Design review of the part built by this model. Coordinates are the model's own, in mm. Face numbers are marked on the shaded views. A direction names the side the tool comes from. Coordinates: 2 decimals unless noted, no trailing zeros. Write each loop counter-clockwise with the first axis right and the second up, starting at its lowest first coordinate (ties: lowest second). Pieces come first, ordered by that corner, then holes. Notation, with made-up numbers: (-38, 5.25) - (4, 5.25) arc R29 ccw to (4, 38.25) - close; hole circle Ø5 at (31, 29.25). An arc over 180 degrees is marked (long way). Use a Markdown table: item, result.
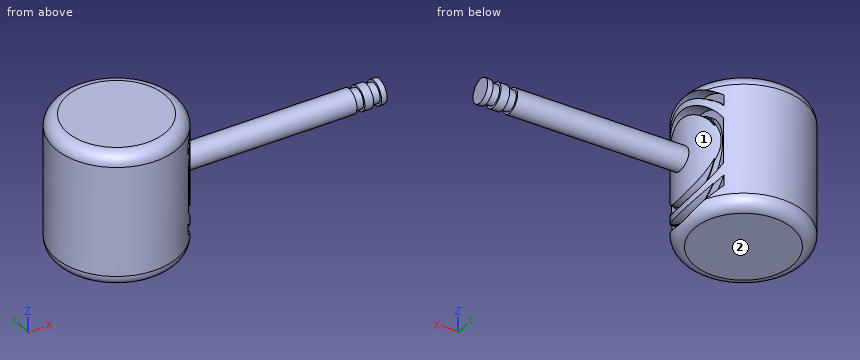
from build123d import *

# Parameters (mm, degrees)
F0_W   = 25.4
F0_H   = 55.7187045847
F2_W   = 118.6923170462
F2_H   = 4.8982012086
F4_W   = 3.185287118
F4_H   = 12.2274383903
F4_W_2 = 20.8224356174
F4_H_2 = 3.0317753553


# Not quite as in the source:
# - a fillet or chamfer that OpenCascade refuses, or shapes differently, is made with other operations: its cross-section is extruded or revolved along the edge and cut away or added


with BuildPart() as f1:
    # F0 (on Front) → F1 (revolve)
    with BuildSketch(Plane.XZ):
        Rectangle(F0_W, F0_H)
    revolve(axis=Axis((12.7, 0, 0), (0, 0, -1)))

    # F2 (on Front) → F3 (revolve)
    with BuildSketch(Plane.XZ):
        with Locations((59.3461585231, -2.4491006043)):
            Rectangle(F2_W, F2_H)
    revolve(axis=Axis((59.3461585231, 0, 0), (-1, 0, 0)))

    # F4 (on Front) → F6 (revolve, cut)
    with BuildSketch(Plane.XZ):
        with Locations((114.8856207728, -10.0567732006)):
            Rectangle(F4_W, F4_H)
        with Locations((108.191460371, -10.1317744702)):
            Rectangle(F4_W, F4_H)
        with Locations((43.9788103104, -24.0039676428)):
            Rectangle(F4_W_2, F4_H_2)
        with Locations((43.7408648431, -17.8672224283)):
            Rectangle(F4_W_2, F4_H_2)
        with Locations((41.584610939, 18.3283146471)):
            Rectangle(F4_W_2, F4_H_2)
        with Locations((41.4398871362, 24.3011359125)):
            Rectangle(F4_W_2, F4_H_2)
    revolve(axis=Axis((52.5897778571, 0, 0), (1, 0, 0)), mode=Mode.SUBTRACT)

    # F7: fillet of radius 5 on 1 edges, made by hand

    # F7_s1 → F7_t2 (revolve, cut)
    with BuildSketch(Plane.XZ):
        with BuildLine():
            ThreePointArc((-12.7, -22.8593522923), (-11.2355339059, -26.3948861983), (-7.7, -27.8593522923))
            Line((-7.7, -27.8593522923), (-12.7, -27.8593522923))
            Line((-12.7, -27.8593522923), (-12.7, -22.8593522923))
        make_face()
    revolve(axis=Axis((12.7, 0, -27.8593522923), (0, 0, -1)), mode=Mode.SUBTRACT)

    # F8: fillet of radius 5 on 1 edges, made by hand

    # F8_s1 → F8_t2 (revolve, cut)
    with BuildSketch(Plane.XZ):
        with BuildLine():
            ThreePointArc((-7.7, 27.8593522923), (-11.2355339059, 26.3948861983), (-12.7, 22.8593522923))
            Line((-12.7, 22.8593522923), (-12.7, 27.8593522923))
            Line((-12.7, 27.8593522923), (-7.7, 27.8593522923))
        make_face()
    revolve(axis=Axis((12.7, 0, 27.8593522923), (0, 0, -1)), mode=Mode.SUBTRACT)


solid = f1.part
(1) Take a section at B-B on x = 50.5. Write out the cut boundary in (y, z), and give its area (3 significant figures).
Determined:
| item | result |
|---|---|
| outline | circle Ø9.8 at (0, 0) |
| area | 75.4 mm2 |
(2) Take a section at A-A on z = 0. Write out the cut boundary in (x, y), and give its area (3 significant figures).
Determined:
| item | result |
|---|---|
| outline | (31.17, -17.43) - (31.17, -16.81) - (31.74, -16.81) arc R25.4 ccw to (37.62, -4.9) - (106.6, -4.9) - (106.6, -4.02) - (109.78, -4.02) - (109.78, -4.9) - (113.29, -4.9) - (113.29, -3.94) - (116.48, -3.94) - (116.48, -4.9) - (118.69, -4.9) - (118.69, 4.9) - (116.48, 4.9) - (116.48, 3.94) - (113.29, 3.94) - (113.29, 4.9) - (109.78, 4.9) - (109.78, 4.02) - (106.6, 4.02) - (106.6, 4.9) - (37.62, 4.9) arc R25.4 ccw to (31.74, 16.81) - (31.17, 16.81) - (31.17, 17.43) arc R25.4 ccw (long way) to start |
| area | 2,810 mm2 |
(3) For pin 1 (3 mm diameter, centred on x = 67, y = -2.5, fed in from -Z); pin 2 (1.7 mm diameter, centred on y = 1, z = -19, fed in from +X); pin 3 (10 mm diameter, centred on x = 69.5, z = 0.5, fed in from +Y), all flat-tipped, find the tip position at first contact; note any pin that passes through.
Determined:
| item | result |
|---|---|
| pin 1 | z = -4.8 |
| pin 2 | x = 38.09 |
| pin 3 | y = 4.9 |
(4) For L1, parallel to X at y = -2.5, z = 4; L2, parallel to Z at x = 32, y = 6; L3, parallel to X at y = 1, z = -20.5, list the stretches that pass through material, from the lowest coordinate up. Write a range as from..to.
Determined:
| item | result |
|---|---|
| L1 | -12.58..106.6, 109.78..113.29, 116.48..118.69 |
| L2 | -27.86..-25.11, -21.98..-18.92, -15.71..15.71, 18.92..21.98, 25.11..27.86 |
| L3 | -12.68..38.08 |
(5) Machinability: for the marked faces 1 and 2, which of the approach directions +Z, -Z, +X, -X, +Y, -Y give a long, thin tool a straight path to every point of the face, cutting with its end or side? Answer none if there is none.
Determined:
| item | result |
|---|---|
| face 1 | +X |
| face 2 | -Z, +X, -X, +Y, -Y |
